Can you work these out from the model? Positions are in its coordinate system, mm. A direction names the side the tool comes from. Give positions to 0.01 mm unless a question says otherwise; leave off trailing zeros. Write each loop counter-clockwise with the first axis right and the second up, starting at its lowest first coordinate (ties: lowest second). Pieces come first, ordered by that corner, then holes. Notation, with made-up numbers: (53, -37) -> (79, -37) arc R13 cw to (79, -30) -> close; hole circle Ø5 at (32.25, 17). An arc over 180 degrees is marked (long way). Answer as CSV lines item,"result". Start each with the question number.
1. If we section it at B-B on x = -11: Write out the boundary of the cut face in (y, z), plus the area to 3 significant figures.
2. If we section it at D-D on y = -7.75: Write out the boundary of the cut face in (x, z).
3. I need wall thicknesses on line 1 (X direction, y = -3.5, z = 1.75); line 2 (Y direction, x = -13, z = -2); line 3 (Z direction, x = -14.75, y = 6.5). Which ranges of each line are inside material? Lowest first, please. Write a range as [from, to].
4. If we mould it in two halves opening along X, with no side actions, what happens to faces 3 (the face through (-20.58, 7.65, 0.02)), 4 (the face through (-21.295, 2.148, -0.021)), 5 (the face through (-9.628, 9.323, 0.021))? For each: pulls with the +X half, pulls with the -X half, needs draft (parallel to the pull), parting line crosses it, or undercut.
5. I'm going to push flat-ended pins straight in: P1, Ø2, axis at x = -10, z = 1.5, coming from the -Y side; P2, Ø0.9, axis at x = -5.5, z = -0.5, coming from the +Y side; P3, Ø3, axis at y = 1.5, z = -1, coming from the -X side. Where does each tip first touch, or does it pass through?
6. On a 3-axis mill with a long thin cutter (end or side, diameter ignored), from which of +Z, -Z, +X, -X, +Y, -Y can I reach the whole of each face in a straight line? I mean faces 1 (the face through (-17, 1, 1.5)), 2 (the face through (-26, -1.86, -0.02)). Say none if no direction works.
7. If we section it at C-C on y = 6.5: Write out the boundary of the cut face in (x, z), plus the area to 3 significant figures.
```python
from build123d import *

# Parameters (mm, degrees)
F0_R     = 5.8
F0_W     = 7.4
F0_H     = 7.4
F1_DEPTH = 3.3
F0_R_2   = 6.5
F2_DEPTH = 1.5
F3_R     = 2
F4_R     = 1
F5_R     = 1
F6_R     = 6.45
F6_R_2   = 5.8
F7_DEPTH = 1.8


with BuildPart() as f1:
    # F0 (on Top) → F1 (new body, symmetric)
    with BuildSketch(Plane.XY):
        with Locations((-11.810101, -3.645376)):
            Circle(F0_R)
        with Locations((-11.810101, -3.645376)):
            Rectangle(F0_W, F0_H, mode=Mode.SUBTRACT)
    extrude(amount=F1_DEPTH, both=True)

    # F0 (on Top) → F2 (join, symmetric)
    with BuildSketch(Plane.XY):
        with BuildLine():
            Line((-22.810101, -13.645376), (-11.810101, -13.645376))
            ThreePointArc((-11.810101, -13.645376), (-4.739033, -10.716444), (-1.810101, -3.645376))
            Line((-1.810101, -3.645376), (-1.810101, 7.354624))
            Line((-1.810101, 7.354624), (-1.810101, 7.854624))
            Line((-1.810101, 7.854624), (-9.43136, 7.854624))
            Line((-9.43136, 7.854624), (-9.814863, 10.716693))
            ThreePointArc((-9.814863, 10.716693), (-11.810101, 10.854624), (-13.805339, 10.716693))
            Line((-13.805339, 10.716693), (-14.293907, 7.070533))
            Line((-14.293907, 7.070533), (-17.631077, 5.688232))
            Line((-17.631077, 5.688232), (-20.554771, 7.920986))
            ThreePointArc((-20.554771, 7.920986), (-22.063149, 6.607672), (-23.376464, 5.099294))
            Line((-23.376464, 5.099294), (-21.143709, 2.175599))
            Line((-21.143709, 2.175599), (-22.52601, -1.16157))
            Line((-22.52601, -1.16157), (-26.17217, -1.650138))
            ThreePointArc((-26.17217, -1.650138), (-26.310101, -3.645376), (-26.17217, -5.640615))
            Line((-26.17217, -5.640615), (-23.310101, -6.024118))
            Line((-23.310101, -6.024118), (-23.310101, -13.645376))
            Line((-23.310101, -13.645376), (-22.810101, -13.645376))
        make_face()
        with Locations((-11.810101, -3.645376)):
            Circle(F0_R_2, mode=Mode.SUBTRACT)
        with Locations((-11.810101, -3.645376)):
            Circle(F0_R_2)
        with Locations((-11.810101, -3.645376)):
            Circle(F0_R, mode=Mode.SUBTRACT)
    extrude(amount=F2_DEPTH, both=True)

    # F3
    f3_edges = [f1.edges().sort_by_distance(p)[0] for p in [
        (-23.310101, -13.645376, 0),
        (-1.810101, 7.854624, 0),
    ]]
    fillet(f3_edges, radius=F3_R)

    # F4
    f4_edges = [f1.edges().sort_by_distance(p)[0] for p in [
        (-26.17217, -5.640615, 0),
        (-26.17217, -1.650138, 0),
        (-23.376464, 5.099294, 0),
        (-20.554771, 7.920986, 0),
        (-13.805339, 10.716693, 0),
        (-9.814863, 10.716693, 0),
    ]]
    fillet(f4_edges, radius=F4_R)

    # F5
    f5_edges = [f1.edges().sort_by_distance(p)[0] for p in [
        (-23.310101, -6.024118, 0),
        (-22.52601, -1.16157, 0),
        (-21.143709, 2.175599, 0),
        (-17.631077, 5.688232, 0),
        (-14.293907, 7.070533, 0),
        (-9.43136, 7.854624, 0),
    ]]
    fillet(f5_edges, radius=F5_R)

    # F6 (on face) → F7 (join, through all)
    with BuildSketch(Plane.XY.offset(1.5)):
        with Locations((-11.810101, -3.645376)):
            Circle(F6_R)
        with Locations((-11.810101, -3.645376)):
            Circle(F6_R_2, mode=Mode.SUBTRACT)
    extrude(amount=F7_DEPTH)


solid = f1.part
```
Computed values:
1,outline,"(-13.61, -1.5) -> (-9.39, -1.5) -> (-9.39, -3.3) -> (-7.35, -3.3) -> (-7.35, 3.3) -> (-10.04, 3.3) -> (-10.04, 1.5) -> (-13.61, 1.5) -> close; (0.05, -3.3) -> (2.1, -3.3) -> (2.1, -1.5) -> (10.83, -1.5) -> (10.83, 1.5) -> (2.75, 1.5) -> (2.75, 3.3) -> (0.05, 3.3) -> close"
1,area,"68.2 mm2"
2,outline,"(-23.31, -1.5) -> (-15.91, -1.5) -> (-15.91, -3.3) -> (-7.71, -3.3) -> (-7.71, -1.5) -> (-2.69, -1.5) -> (-2.69, 1.5) -> (-6.83, 1.5) -> (-6.83, 3.3) -> (-16.79, 3.3) -> (-16.79, 1.5) -> (-23.31, 1.5) -> close"
3,line 1,"x = [-18.26, -15.51], [-8.11, -5.36]"
3,line 2,"y = [-9.32, -7.35], [0.05, 2.03]"
3,line 3,"z = [-1.5, 1.5]"
4,face 3,"undercut"
4,face 4,"pulls with the -X half"
4,face 5,"pulls with the +X half"
5,P1,"stops at y = -13.61"
5,P2,"stops at y = 7.85"
5,P3,"stops at x = -22.04"
6,face 1,"+Z"
6,face 2,"+Z, -Z, -X, +Y"
7,outline,"(-22.17, -1.5) -> (-18.69, -1.5) -> (-18.69, 1.5) -> (-22.17, 1.5) -> close; (-15.67, -1.5) -> (-1.92, -1.5) -> (-1.92, 1.5) -> (-15.67, 1.5) -> close"
7,area,"51.7 mm2"
